Input: part model. Units: mm. Frame: model coordinates. Face numbers are marked on the shaded views. A direction names the side the tool comes from. Give positions to 0.01 mm unless a question says otherwise; leave off trailing zeros. Loops run counter-clockwise (first coordinate to the right, second up) from the corner with the lowest first, then second, coordinate; pieces in that order, holes last. Notation, with made-up numbers: (-28.75, -8.75) -> (6.25, -8.75) arc R14 cw to (6.25, 8.25) -> close; hole circle Ø4 at (-29, 43.5). An arc over 180 degrees is marked (long way). Answer as a JSON object with one key per item and string values.
```python
from build123d import *

# Parameters (mm, degrees)
F0_W     = 3
F0_H     = 7
F0_H_2   = 2
F0_H_3   = 16
F2_ANGLE = 180


# Not quite as in the source:
# - a feature names something its author has since deleted; it is built from what else it names


with BuildPart() as f1:
    # F0 (on Front) → F1 (revolve)
    with BuildSketch(Plane.XZ):
        Polygon((0, 14.5), (0, 12.5), (3, 12.5), (3, 10.5), (11, 10.5), (11, 14.5), align=None)
        with Locations((1.5, 7)):
            Rectangle(F0_W, F0_H)
        with Locations((1.5, 11.5)):
            Rectangle(F0_W, F0_H_2)
        with Locations((1.5, -4.5)):
            Rectangle(F0_W, F0_H_3)
    revolve(axis=Axis((0, 0, 1), (0, 0, -1)))

    # F0 (on Front) → F2 (revolve, cut)
    with BuildSketch(Plane.XZ):
        with Locations((-1.5, -4.5)):
            Rectangle(F0_W, F0_H_3)
    revolve(axis=Axis((0, 0, 1), (0, 0, 1)), revolution_arc=F2_ANGLE, mode=Mode.SUBTRACT)


solid = f1.part
```
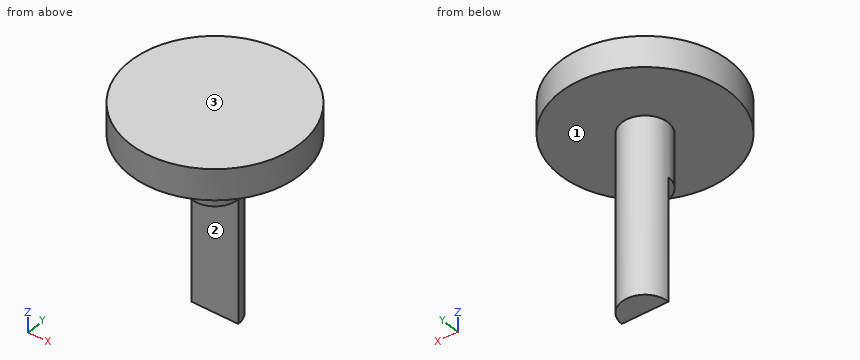
Q1. Section A-A, the plane x = 0. Return the cut outline in (y, z), then the cut area to 3 significant figures.
Evaluation:
{"outline": "(-11, 10.5) -> (-3, 10.5) -> (-3, 3.5) -> (0, 3.5) -> (0, -12.5) -> (3, -12.5) -> (3, 10.5) -> (11, 10.5) -> (11, 14.5) -> (-11, 14.5) -> close", "area": "178 mm2"}
Q2. Access query for the marked faces 1, 2 and 3. Directions: +Z, -Z, +X, -X, +Y, -Y. A direction counts if a zero-diameter tool reaches every point of the face in a straight line with its end or side. Return the directions, or none.
Evaluation:
{"face 1": "-Z", "face 2": "-Z, +X, -X, -Y", "face 3": "+Z, +X, -X, +Y, -Y"}
Q3. Section B-B, the plane z = -8.75. Return the cut outline in (x, y).
Evaluation:
{"outline": "(-3, 0) -> (3, 0) arc R3 ccw to start"}
Q4. Section C-C, the plane y = -2. Return the cut outline in (x, z), then the cut area to 3 significant figures.
Evaluation:
{"outline": "(-10.82, 10.5) -> (-2.24, 10.5) -> (-2.24, 3.5) -> (2.24, 3.5) -> (2.24, 10.5) -> (10.82, 10.5) -> (10.82, 14.5) -> (-10.82, 14.5) -> close", "area": "118 mm2"}
Q5. Section D-D, the plane y = 5.25. Return the cut outline in (x, z), then the cut area to 3 significant figures.
Evaluation:
{"outline": "(-9.67, 10.5) -> (9.67, 10.5) -> (9.67, 14.5) -> (-9.67, 14.5) -> close", "area": "77.3 mm2"}
Q6. Pin query (flat end, axial travel): pin 1 (10 mm diameter, centred on x = -4.5, y = -6.5, fed in from -Z); pin 2 (6 mm diameter, centred on x = 7.5, y = 7.5, fed in from -Z); pin 3 (6.5 mm diameter, centred on x = 0, z = -1.5, fed in from -Y). Return the tip coordinate at first contact, or that it passes through.
Evaluation:
{"pin 1": "stops at z = 3.5", "pin 2": "stops at z = 10.5", "pin 3": "stops at y = 0"}
Q7. Ray query, line 1 along Z through (x, y) = (4.75, -6.5); line 2 along X through (y, z) = (1, 12); line 3 along Y through (x, z) = (-1, -7). Return the intervals inside material, ascending.
Evaluation:
{"line 1": "z = 10.5 to 14.5", "line 2": "x = -10.95 to 10.95", "line 3": "y = 0 to 2.83"}
